from build123d import *

# Parameters (mm, degrees)
SKETCH1_R           = 43.5
SKETCH1_R_2         = 38.5
BOSS_EXTRUDE3_DEPTH = 95
SKETCH3_R           = 53.5
BOSS_EXTRUDE4_DEPTH = 5
SKETCH4_R           = 38.5
CUT_EXTRUDE1_DEPTH  = 5
SKETCH5_R           = 39
CUT_EXTRUDE2_DEPTH  = 120
SKETCH6_R           = 43.5
CUT_EXTRUDE3_DEPTH  = 3


with BuildPart() as part:
    # Sketch1 → Boss-Extrude3 (new body)
    with BuildSketch(Plane(origin=(0, 0, 0), x_dir=(1, 0, 0), z_dir=(0, 1, 0))):
        with Locations(Location((0, 0, 0), (0, 0, 270))):
            Circle(SKETCH1_R)
        with Locations(Location((0, 0, 0), (0, 0, 270))):
            Circle(SKETCH1_R_2, mode=Mode.SUBTRACT)
    extrude(amount=BOSS_EXTRUDE3_DEPTH)

    # Sketch3 → Boss-Extrude4 (add)
    with BuildSketch(Plane(origin=(0, 95, 0), x_dir=(1, 0, 0), z_dir=(0, 1, 0))):
        with Locations(Location((0, 0, 0), (0, 0, 270))):
            Circle(SKETCH3_R)
    extrude(amount=BOSS_EXTRUDE4_DEPTH)

    # Sketch4 → Cut-Extrude1 (cut)
    with BuildSketch(Plane.XZ.offset(-95)):
        with Locations(Location((0, 0, 0), (0, 0, 270))):
            Circle(SKETCH4_R)
    extrude(amount=-CUT_EXTRUDE1_DEPTH, mode=Mode.SUBTRACT)

    # Sketch5 → Cut-Extrude2 (cut)
    with BuildSketch(Plane(origin=(0, 100, 0), x_dir=(1, 0, 0), z_dir=(0, 1, 0))):
        with Locations(Location((0, 0, 0), (0, 0, 270))):
            Circle(SKETCH5_R)
    extrude(amount=-CUT_EXTRUDE2_DEPTH, mode=Mode.SUBTRACT)

    # Sketch6 → Cut-Extrude3 (cut)
    with BuildSketch(Plane.XZ):
        with Locations(Location((0, 0, 0), (0, 0, 270))):
            Circle(SKETCH6_R)
    extrude(amount=-CUT_EXTRUDE3_DEPTH, mode=Mode.SUBTRACT)


solid = part.part
Part model, mm, in its own coordinate system. Give positions to 0.01 mm unless a question says otherwise; leave off trailing zeros. Order: outer loops, then holes, each group sorted by start corner. A loop starts at its lowest first (then second) coordinate and runs counter-clockwise, first axis right, second up. Notation, with made-up numbers: (-25, 27) - (-10, 27) arc R22 cw to (-10, 45) - close; hole circle Ø8 at (81.5, 25.25). An arc over 180 degrees is marked (long way). One line per question, with ' | ' between items.
1. Band-saw the part on D-D on x = -41.5. List the corners of the cut face in (y, z), then the cut area to 3 significant figures.
Filled in:
outline: (3, -13.04) - (95, -13.04) - (95, -33.76) - (100, -33.76) - (100, 33.76) - (95, 33.76) - (95, 13.04) - (3, 13.04) - close | area: 2,740 mm²
2. Band-saw the part on A-A on z = 0. List the corners of the cut face in (x, y).
Filled in:
outline: (-53.5, 95) - (-43.5, 95) - (-43.5, 3) - (-39, 3) - (-39, 100) - (-53.5, 100) - close; (39, 3) - (43.5, 3) - (43.5, 95) - (53.5, 95) - (53.5, 100) - (39, 100) - close
3. Band-saw the part on C-C on y = 23.5. List the corners of the cut face in (x, z), then the cut area to 3 significant figures.
Filled in:
outline: circle Ø87 at (0, 0); hole circle Ø78 at (0, 0) | area: 1,170 mm²
4. Band-saw the part on B-B on x = 0. List the corners of the cut face in (y, z), then the cut area to 3 significant figures.
Filled in:
outline: (3, -43.5) - (95, -43.5) - (95, -53.5) - (100, -53.5) - (100, -39) - (3, -39) - close; (3, 39) - (100, 39) - (100, 53.5) - (95, 53.5) - (95, 43.5) - (3, 43.5) - close | area: 973 mm²
5. Pull direction Z, two halves, no side cores. Call faces 1 (the face through (43.13, 48.36, -5.66)), 2 (the face through (38.668, 52.179, -5.077)), 3 (the face through (44, 95, 0)): +Z half, -Z half, draft (parallel to the pull), parting line (faces both ways), or undercut.
Filled in:
face 1: parting line | face 2: undercut | face 3: draft
6. Drill centre lines: probe 1 along X at (y, z) = (69, 0); probe 2 along Y at (x, z) = (21.5, 47.5); probe 3 along X at (y, z) = (48, -25.5). Where is each one in solid material? Low to high.
Filled in:
probe 1: -43.5 to -39, 39 to 43.5 | probe 2: 95 to 100 | probe 3: -35.24 to -29.51, 29.51 to 35.24
7. Drop flat-ended pins along their axis: P1, Ø2, axis at x = 6.5, y = 83, coming from the +Z side; P2, Ø6, axis at y = 39.5, z = 25, coming from the +X side; P3, Ø6, axis at x = 14, y = 26, coming from the -Z side; P4, Ø12, axis at x = 32, z = 2.5, coming from the -Y side. Give the stop position or say it passes through.
Filled in:
P1: z = 43.15 | P2: x = 37.53 | P3: z = -42.09 | P4: through
